For this review, use the dimensioned drawing (mm, ordinates from the lowest corner) and the shaded views. A direction names the side the tool comes from. Round coordinates to 2 decimals unless told otherwise and drop trailing zeros. Order: outer loops, then holes, each group sorted by start corner. A loop starts at its lowest first (then second) coordinate and runs counter-clockwise, first axis right, second up. Notation, with made-up numbers: (-0.5, 67.5) -> (53.5, 67.5) arc R19 cw to (53.5, 90.5) -> close; hole circle Ø4 at (14.5, 3.25). An arc over 180 degrees is marked (long way). Answer in a Markdown table with one row per item.
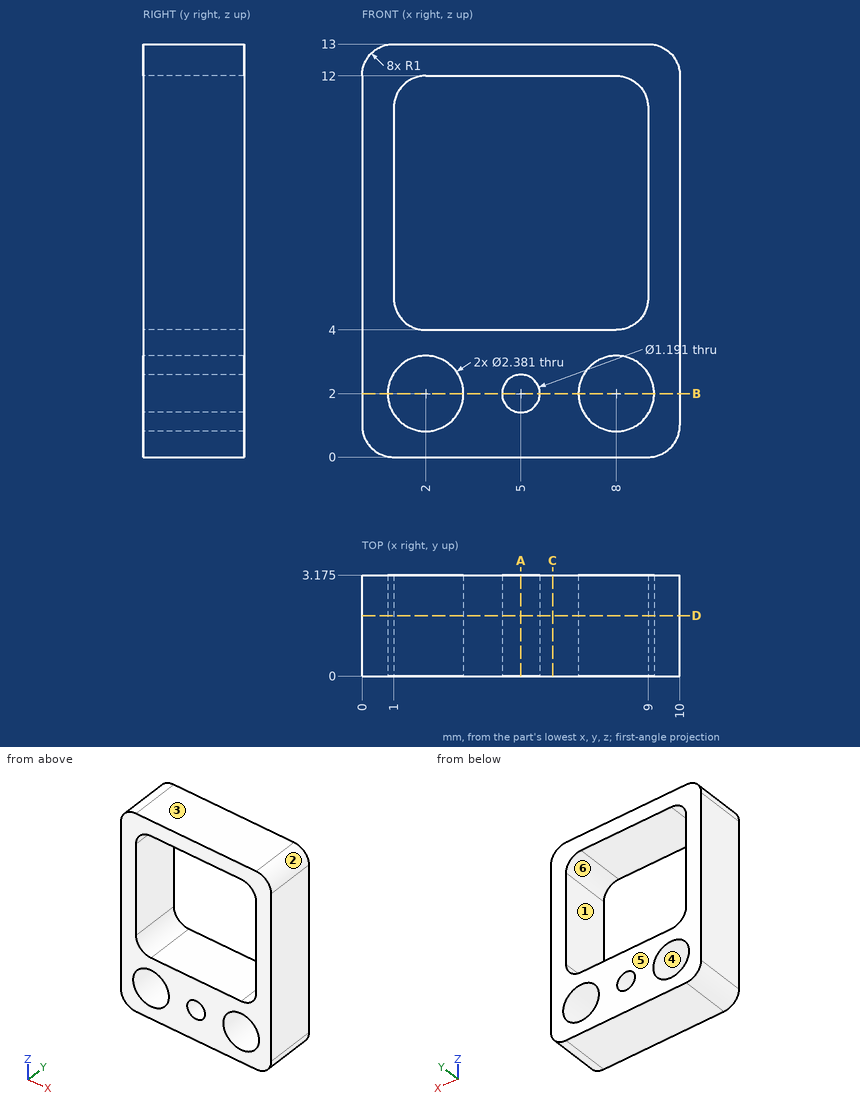
Q1. Tool access review of the marked faces 1 and 2: name each direction out of +Z, -Z, +X, -X, +Y, -Y from which nothing blocks a thin tool from reaching the whole face with its end or side.
Answer key:
| item | result |
|---|---|
| face 1 | +Y, -Y |
| face 2 | +Z, +X, +Y, -Y |
Q2. To check wall thickness, follow probe 1 along X at (y, z) = (1.05, 2); probe 2 along Z at (x, y) = (5.75, 3.05); probe 3 along X at (y, z) = (0.75, 10). State the ranges of each line that lie inside material, in increasing order.
Answer key:
| item | result |
|---|---|
| probe 1 | x = 0 to 0.81, 3.19 to 4.4, 5.6 to 6.81, 9.19 to 10 |
| probe 2 | z = 0 to 4, 12 to 13 |
| probe 3 | x = 0 to 1, 9 to 10 |
Q3. Take a section at D-D, the plane y = 1.9. Write out the cut boundary in (x, z).
Answer key:
| item | result |
|---|---|
| outline | (0, 1) arc R1 ccw to (1, 0) -> (9, 0) arc R1 ccw to (10, 1) -> (10, 12) arc R1 ccw to (9, 13) -> (1, 13) arc R1 ccw to (0, 12) -> close; hole circle Ø2.38 at (2, 2); hole (1, 5) arc R1 ccw to (2, 4) -> (8, 4) arc R1 ccw to (9, 5) -> (9, 11) arc R1 ccw to (8, 12) -> (2, 12) arc R1 ccw to (1, 11) -> close; hole circle Ø1.19 at (5, 2); hole circle Ø2.38 at (8, 2) |
Q4. Take a section at C-C, the plane x = 6. Write out the cut boundary in (y, z) (1 decimal).
Answer key:
| item | result |
|---|---|
| outline | (0, 0) -> (3.2, 0) -> (3.2, 4) -> (0, 4) -> close; (0, 12) -> (3.2, 12) -> (3.2, 13) -> (0, 13) -> close |
Q5. Take a section at A-A, the plane x = 5. Write out the cut boundary in (y, z) (1 decimal).
Answer key:
| item | result |
|---|---|
| outline | (0, 0) -> (3.2, 0) -> (3.2, 1.4) -> (0, 1.4) -> close; (0, 2.6) -> (3.2, 2.6) -> (3.2, 4) -> (0, 4) -> close; (0, 12) -> (3.2, 12) -> (3.2, 13) -> (0, 13) -> close |
Q6. Clearance check with a flat-ended pin moving along its axis: pin 1 Ø1 at (y, z) = (2, 7.5) entering from -X. State where the tip first meets the part, or that it passes through.
Answer key:
| item | result |
|---|---|
| pin 1 | stops at x = 0 |
Q7. The part is to be moulded in two halves that separate along Z. For the marked faces 3, 4, 5 and 6, say which applies: +Z half, -Z half, draft (parallel to the pull), parting line (faces both ways), or undercut.
Answer key:
| item | result |
|---|---|
| face 3 | +Z half |
| face 4 | undercut |
| face 5 | draft |
| face 6 | undercut |
Q8. Take a section at B-B, the plane z = 2. Write out the cut boundary in (x, y) (1 decimal).
Answer key:
| item | result |
|---|---|
| outline | (0, 0) -> (0.8, 0) -> (0.8, 3.2) -> (0, 3.2) -> close; (3.2, 0) -> (4.4, 0) -> (4.4, 3.2) -> (3.2, 3.2) -> close; (5.6, 0) -> (6.8, 0) -> (6.8, 3.2) -> (5.6, 3.2) -> close; (9.2, 0) -> (10, 0) -> (10, 3.2) -> (9.2, 3.2) -> close |
